Verification items for the finished model (mm, model axes). Face numbers are marked on the shaded views. A direction names the side the tool comes from. Round coordinates to 2 decimals unless told otherwise and drop trailing zeros. Write each loop counter-clockwise with the first axis right and the second up, starting at its lowest first coordinate (ties: lowest second). Pieces come first, ordered by that corner, then holes. Notation, with made-up numbers: M 62.25,43.5 L 97.25,43.5 A33 cw 97.25,74.5 Z; hole C 78,5 d8. An arc over 180 degrees is marked long. Answer in a Markdown table with one row per item. Add a question column.
1. Sectioned sample at A-A on x = -7. Record the cut outline in (y, z), plus the area to 3 significant figures.
2. Material ranges on probe 1 along X at (y, z) = (0, 16.9); probe 2 along X at (y, z) = (10.25, -13.55); probe 3 along X at (y, z) = (0, -16.8), recorded low to high.
3. Draft check along X on the marked faces 1, 2, 3 and 4. Enter one of: pulls with the +X half, pulls with the -X half, needs draft (parallel to the pull), parting line crosses it, or undercut.
4. Set-up check for the marked faces 5, 6, 7, 8 and 9: record each of +Z, -Z, +X, -X, +Y, -Y from which the full face is reachable in a straight line by a thin tool's end or side.
5. Sectioned sample at D-D on x = 13. Record the cut outline in (y, z), plus the area to 3 significant figures.
6. Sectioned sample at B-B on y = -4.25. Record the cut outline in (x, z).
7. Sectioned sample at C-C on x = 32.75. Record the cut outline in (y, z).
8. Go/stop test with flat-tipped pins: pin 1 Ø0.7 at (y, z) = (-1, -17.5) entering from +X; pin 2 Ø3 at (x, z) = (13.5, 16) entering from +Y; pin 3 Ø10 at (x, y) = (24.5, 7.5) entering from +Z; pin 4 Ø0.8 at (x, z) = (27, 16.5) entering from +Y. Record where each tip stops, or that it passes through.
```python
from build123d import *

# Parameters (mm, degrees)
S_BOX1_W      = 45.4
S_BOX1_H      = 24.8
BOSS_1_DEPTH  = 30.3
S_BOX2_W      = 29.9
S_BOX2_H      = 24.8
BOSS_2_DEPTH  = 1.3
S_BOX3_W      = 13.2
S_BOX3_H      = 18.4
BOSS_3_DEPTH  = 2.35
S_CYL4_R      = 3
BOSS_4_DEPTH  = 4.05
S_BOX5_W      = 26.4
S_BOX5_H      = 14
BOSS_5_DEPTH  = 1.65
S_CYL6_R      = 5.3
BOSS_6_DEPTH  = 0.6
S_CYL7_R      = 10
BOSS_7_DEPTH  = 2.2
S_CYL8_R      = 10
BOSS_8_DEPTH  = 2.95
S_CYL9_R      = 2.8
BOSS_9_DEPTH  = 1.65
S_HOLE10_R    = 1.25
HOLE_10_DEPTH = 2.25
S_HOLE11_R    = 1.25
HOLE_11_DEPTH = 2.25
S_HOLE12_R    = 1.25
HOLE_12_DEPTH = 2.25
S_HOLE13_R    = 1.25
HOLE_13_DEPTH = 2.25
S_HOLE14_R    = 1.25
HOLE_14_DEPTH = 2.6
S_HOLE15_R    = 1.25
HOLE_15_DEPTH = 2.6
S_HOLE16_R    = 1.25
HOLE_16_DEPTH = 2.6
S_HOLE17_R    = 1.25
HOLE_17_DEPTH = 2.6
S_HOLE18_R    = 0.8
HOLE_18_DEPTH = 3
S_HOLE19_R    = 0.8
HOLE_19_DEPTH = 3
S_HOLE20_R    = 0.8
HOLE_20_DEPTH = 3
S_HOLE21_R    = 0.8
HOLE_21_DEPTH = 3


with BuildPart() as part:
    # S_box1 → Boss_1 (new body)
    with BuildSketch(Plane.XY.offset(-14.4)):
        with Locations((12.5, 0)):
            Rectangle(S_BOX1_W, S_BOX1_H)
    extrude(amount=BOSS_1_DEPTH)

    # S_box2 → Boss_2 (add)
    with BuildSketch(Plane.XY.offset(-15.6)):
        with Locations((20.25, 0)):
            Rectangle(S_BOX2_W, S_BOX2_H)
    extrude(amount=BOSS_2_DEPTH)

    # S_box3 → Boss_3 (add)
    with BuildSketch(Plane.XY.offset(-17.85)):
        with Locations((23.3, 0)):
            Rectangle(S_BOX3_W, S_BOX3_H)
    extrude(amount=BOSS_3_DEPTH)

    # S_cyl4 → Boss_4 (add)
    with BuildSketch(Plane.XY.offset(-18.35)):
        Circle(S_CYL4_R)
    extrude(amount=BOSS_4_DEPTH)

    # S_box5 → Boss_5 (add)
    with BuildSketch(Plane.XY.offset(15.8)):
        with Locations((21.8, 0)):
            Rectangle(S_BOX5_W, S_BOX5_H)
    extrude(amount=BOSS_5_DEPTH)

    # S_cyl6 → Boss_6 (add)
    with BuildSketch(Plane.XY.offset(15.8)):
        with Locations(Location((0, 0, 0), (0, 0, 180))):
            Circle(S_CYL6_R)
    extrude(amount=BOSS_6_DEPTH)

    # S_cyl7 → Boss_7 (add)
    with BuildSketch(Plane.XY.offset(-17.75)):
        with Locations(Location((0, 0, 0), (0, 0, 302.005454828))):
            Circle(S_CYL7_R)
    extrude(amount=BOSS_7_DEPTH)

    # S_cyl8 → Boss_8 (add)
    with BuildSketch(Plane.XY.offset(15.8)):
        with Locations(Location((0, 0, 0), (0, 0, 302.005454828))):
            Circle(S_CYL8_R)
    extrude(amount=BOSS_8_DEPTH)

    # S_cyl9 → Boss_9 (add)
    with BuildSketch(Plane.XY.offset(18.65)):
        Circle(S_CYL9_R)
    extrude(amount=BOSS_9_DEPTH)

    # S_hole10 → Hole_10 (cut)
    with BuildSketch(Plane.XY.offset(-17.85)):
        with Locations((7, 0)):
            Circle(S_HOLE10_R)
    extrude(amount=HOLE_10_DEPTH, mode=Mode.SUBTRACT)

    # S_hole11 → Hole_11 (cut)
    with BuildSketch(Plane.XY.offset(-17.85)):
        with Locations((0, 7)):
            Circle(S_HOLE11_R)
    extrude(amount=HOLE_11_DEPTH, mode=Mode.SUBTRACT)

    # S_hole12 → Hole_12 (cut)
    with BuildSketch(Plane.XY.offset(-17.85)):
        with Locations((-7, 0)):
            Circle(S_HOLE12_R)
    extrude(amount=HOLE_12_DEPTH, mode=Mode.SUBTRACT)

    # S_hole13 → Hole_13 (cut)
    with BuildSketch(Plane.XY.offset(-17.85)):
        with Locations((0, -7)):
            Circle(S_HOLE13_R)
    extrude(amount=HOLE_13_DEPTH, mode=Mode.SUBTRACT)

    # S_hole14 → Hole_14 (cut)
    with BuildSketch(Plane.XY.offset(16.25)):
        with Locations((7, 0)):
            Circle(S_HOLE14_R)
    extrude(amount=HOLE_14_DEPTH, mode=Mode.SUBTRACT)

    # S_hole15 → Hole_15 (cut)
    with BuildSketch(Plane.XY.offset(16.25)):
        with Locations((0, 7)):
            Circle(S_HOLE15_R)
    extrude(amount=HOLE_15_DEPTH, mode=Mode.SUBTRACT)

    # S_hole16 → Hole_16 (cut)
    with BuildSketch(Plane.XY.offset(16.25)):
        with Locations((-7, 0)):
            Circle(S_HOLE16_R)
    extrude(amount=HOLE_16_DEPTH, mode=Mode.SUBTRACT)

    # S_hole17 → Hole_17 (cut)
    with BuildSketch(Plane.XY.offset(16.25)):
        with Locations((0, -7)):
            Circle(S_HOLE17_R)
    extrude(amount=HOLE_17_DEPTH, mode=Mode.SUBTRACT)

    # S_hole18 → Hole_18 (cut)
    with BuildSketch(Plane.XY.offset(-15.7)):
        with Locations((8.3, -10.25)):
            Circle(S_HOLE18_R)
    extrude(amount=HOLE_18_DEPTH, mode=Mode.SUBTRACT)

    # S_hole19 → Hole_19 (cut)
    with BuildSketch(Plane.XY.offset(-15.7)):
        with Locations((8.3, 10.25)):
            Circle(S_HOLE19_R)
    extrude(amount=HOLE_19_DEPTH, mode=Mode.SUBTRACT)

    # S_hole20 → Hole_20 (cut)
    with BuildSketch(Plane.XY.offset(-15.7)):
        with Locations((32.75, -10.25)):
            Circle(S_HOLE20_R)
    extrude(amount=HOLE_20_DEPTH, mode=Mode.SUBTRACT)

    # S_hole21 → Hole_21 (cut)
    with BuildSketch(Plane.XY.offset(-15.7)):
        with Locations((32.75, 10.25)):
            Circle(S_HOLE21_R)
    extrude(amount=HOLE_21_DEPTH, mode=Mode.SUBTRACT)


solid = part.part
```
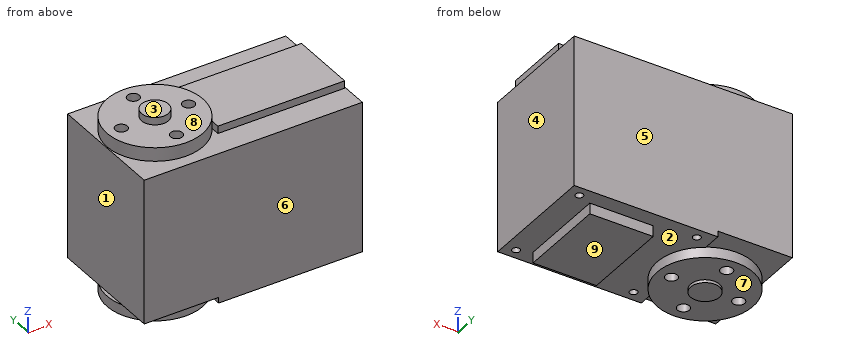
Geometry check:
| question | item | result |
|---|---|---|
| 1 | outline | M -12.4,-14.4 L 12.4,-14.4 L 12.4,15.9 L 7.14,15.9 L 7.14,18.75 L 1.25,18.75 L 1.25,16.25 L -1.25,16.25 L -1.25,18.75 L -7.14,18.75 L -7.14,15.9 L -12.4,15.9 Z; M -7.14,-17.75 L -1.25,-17.75 L -1.25,-15.6 L 1.25,-15.6 L 1.25,-17.75 L 7.14,-17.75 L 7.14,-15.55 L -7.14,-15.55 Z |
| 1 | area | 812 mm2 |
| 2 | probe 1 | x = -10 to -8.25, -5.75 to 5.75, 8.25 to 35 |
| 2 | probe 2 | x = -10.2 to 7.5, 9.1 to 31.95, 33.55 to 35.2 |
| 2 | probe 3 | x = -10 to -8.25, -5.75 to 5.75, 8.25 to 10, 16.7 to 29.9 |
| 3 | face 1 | pulls with the -X half |
| 3 | face 2 | undercut |
| 3 | face 3 | needs draft |
| 3 | face 4 | pulls with the +X half |
| 4 | face 5 | +Z, -Z, +X, -X, +Y |
| 4 | face 6 | +Z, -Z, +X, -X, -Y |
| 4 | face 7 | -Z |
| 4 | face 8 | +Z |
| 4 | face 9 | -Z, +X, +Y, -Y |
| 5 | outline | M -12.4,-15.6 L 12.4,-15.6 L 12.4,15.9 L 7,15.9 L 7,17.45 L -7,17.45 L -7,15.9 L -12.4,15.9 Z |
| 5 | area | 803 mm2 |
| 6 | outline | M -10.2,-14.4 L 5.3,-14.4 L 5.3,-15.55 L -9.05,-15.55 L -9.05,-17.75 L 9.05,-17.75 L 9.05,-15.6 L 16.7,-15.6 L 16.7,-17.85 L 29.9,-17.85 L 29.9,-15.6 L 35.2,-15.6 L 35.2,15.9 L 35,15.9 L 35,17.45 L 9.05,17.45 L 9.05,18.75 L -9.05,18.75 L -9.05,15.9 L -10.2,15.9 Z |
| 7 | outline | M -12.4,-15.6 L -11.05,-15.6 L -11.05,-12.7 L -9.45,-12.7 L -9.45,-15.6 L 9.45,-15.6 L 9.45,-12.7 L 11.05,-12.7 L 11.05,-15.6 L 12.4,-15.6 L 12.4,15.9 L 7,15.9 L 7,17.45 L -7,17.45 L -7,15.9 L -12.4,15.9 Z |
| 8 | pin 1 | stops at x = 29.9 |
| 8 | pin 2 | stops at y = 12.4 |
| 8 | pin 3 | stops at z = 17.45 |
| 8 | pin 4 | stops at y = 7 |
